Geometry check sheet. Reference: the model listing, model coordinates, mm. Face numbers are marked on the shaded views. A direction names the side the tool comes from. Round coordinates to 2 decimals unless told otherwise and drop trailing zeros. Order: outer loops, then holes, each group sorted by start corner. A loop starts at its lowest first (then second) coordinate and runs counter-clockwise, first axis right, second up.
Autodesk Inventor part; units mm, degrees
ref_plane "Work Plane1" through (-20.5858, -18.5858, -56) normal (0, 0, -1) x (0, 1, 0)
ref_plane "YZ Plane" through (0, 0, 0) normal (1, 0, 0) x (0, 1, 0)
ref_plane "XZ Plane" through (0, 0, 0) normal (0, 1, 0) x (-1, 0, 0)
sketch "Base" plane through (0, 0, 0) normal (0, 0, 1) x (1, 0, 0)
  circle A0 centre (0, 0) radius 11 construction
  line L0 (18, 21) -> (-22, 21) construction
  line L1 (-22, -21) -> (18, -21) construction
  line L2 (19, -20) -> (19, 20) construction
  line L3 (-23, 20) -> (-23, -20) construction
  circle A1 centre (0, 0) radius 11.075
  line L4 (-197.84, 0) -> (55.14, 0) construction
  line L5 (-23, 23.05) -> (19, 23.05)
  line L6 (19, 23.05) -> (19, 21.05)
  line L7 (19, 21.05) -> (-23, 21.05)
  line L8 (-23, 21.05) -> (-23, 23.05)
  line L9 (-23, 21.05) -> (19, 21.05)
  line L10 (19, 21.05) -> (19, 0)
  line L11 (19, 0) -> (-23, 0)
  line L12 (-23, 0) -> (-23, 21.05)
  line L13 (-23, -23.05) -> (19, -23.05)
  line L14 (19, -23.05) -> (19, -21.05)
  line L15 (19, -21.05) -> (-23, -21.05)
  line L16 (-23, -21.05) -> (-23, -23.05)
  line L17 (19, -21.05) -> (19, 0)
  line L18 (-23, 0) -> (-23, -21.05)
  line L19 (0, 14) -> (0, 0) construction
  line L20 (0, 0) -> (0, -14) construction
  circle A2 centre (12.3744, -12.3744) radius 1.621
  circle A3 centre (12.3744, 12.3744) radius 1.621
  circle A4 centre (-12.3744, 12.3744) radius 1.621
  circle A5 centre (-12.3744, -12.3744) radius 1.621
  dimension "d0" = 22.15
  dimension "d1" = 2
  dimension "d4" = 0.05
extrude "BaseFeature" add sketch "Base" along normal blind 4 contours L11 L17 L15 L18 A1 | A1 L11 L12 L7 L10 | L7 L8 L5 L6 | L14 L13 L16 L15
ref_plane "Work Plane1" through (-20.5858, -18.5858, -56) normal (0, 0, -1) x (0, 1, 0)
sketch "Sides" plane through (0, 0, 0) normal (0, 0, -1) x (-1, 0, 0)
  line L0 (23, -23.05) -> (-19, -23.05)
  line L1 (-19, -23.05) -> (23, -23.05)
  line L2 (23, -23.05) -> (23, -21.05)
  line L3 (23, -21.05) -> (-19, -21.05)
  line L4 (-19, -21.05) -> (-19, -23.05)
  line L5 (-19, 23.05) -> (23, 23.05)
  line L6 (-19, 23.05) -> (23, 23.05)
  line L7 (23, 23.05) -> (23, 21.05)
  line L8 (23, 21.05) -> (-19, 21.05)
  line L9 (-19, 21.05) -> (-19, 23.05)
  point P0 (0, 0)
extrude "Extrusion2" add sketch "Sides" along normal blind 8
sketch "Sketch3" plane through (-23, -23.05, 4) normal (0, -1, 0) x (1, 0, 0)
  line L0 (42, -12) -> (42, 0)
  line L1 (0, 0) -> (42, 0)
  line L2 (0, -12) -> (0, 0)
  line L3 (42, -12) -> (0, -12)
  point P0 (23, -4)
extrude "Extrusion3" add sketch "Sketch3" along normal blind 1
mirror "Mirror1" about plane through (0, 0, 0) normal (0, 1, 0) of "Extrusion3"
sketch "Sketch4" plane through (-23, -24.05, 4) normal (0, -1, 0) x (1, 0, 0)
  line L0 (0, 0) -> (0, -12) construction
  line L1 (42, -4) -> (42, -12) construction
  circle A0 centre (5.5, -7.5) radius 1.621
  line L2 (21, 0) -> (21, -12) construction
  line L3 (0, -12) -> (42, -12) construction
  line L4 (42, 0) -> (0, 0) construction
  circle A1 centre (36.5, -7.5) radius 1.621
  point P0 (23, -4)
  dimension "d9" = 3.242
  dimension "d15" = 5.5
  dimension "d16" = 4.5
extrude "Extrusion4" cut sketch "Sketch4" against normal through all
chamfer "Chamfer1" distance 2 angle 45 4 edges at (19, 24.05, -2) (-23, 24.05, -2) (19, -24.05, -2) (-23, -24.05, -2)
properties part number "MotorMount"
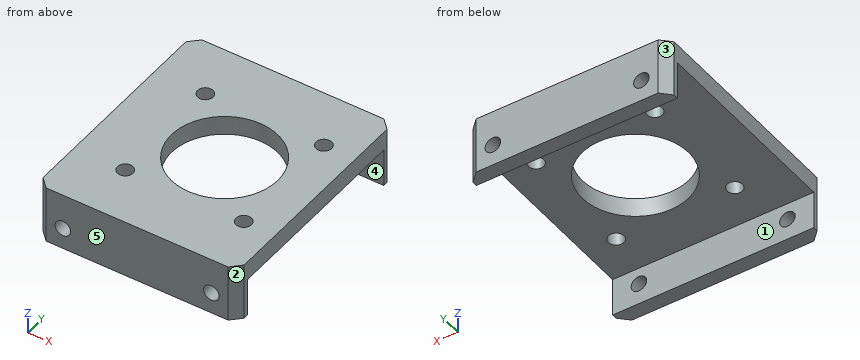
(1) Material ranges on line 1 (Z direction, x = 13.5, y = 22.5); line 2 (Y direction, x = -5, z = -6); line 3 (Z direction, x = 11, y = 9.5), recorded low to high.
Returned:
line 1: z = -8 to -5.12, -1.88 to 4
line 2: y = -24.05 to -21.05, 21.05 to 24.05
line 3: z = 0 to 4
(2) Sectioned sample at A-A, the plane z = -3.5. Record the cut outline in (x, y), and give its area (3 significant figures).
Returned:
outline: (-23, -22.05) - (-21, -24.05) - (-19.12, -24.05) - (-19.12, -21.05) - (-23, -21.05) - close; (-23, 21.05) - (-19.12, 21.05) - (-19.12, 24.05) - (-21, 24.05) - (-23, 22.05) - close; (-15.88, -24.05) - (11.88, -24.05) - (11.88, -21.05) - (-15.88, -21.05) - close; (-15.88, 21.05) - (11.88, 21.05) - (11.88, 24.05) - (-15.88, 24.05) - close; (15.12, -24.05) - (17, -24.05) - (19, -22.05) - (19, -21.05) - (15.12, -21.05) - close; (15.12, 21.05) - (19, 21.05) - (19, 22.05) - (17, 24.05) - (15.12, 24.05) - close
area: 205 mm2
(3) Sectioned sample at D-D, the plane x = -17. Record the cut outline in (y, z).
Returned:
outline: (-24.05, -8) - (-21.05, -8) - (-21.05, -5.04) - (-24.05, -5.04) - close; (-24.05, -1.96) - (-21.05, -1.96) - (-21.05, 0) - (21.05, 0) - (21.05, -1.96) - (24.05, -1.96) - (24.05, 4) - (-24.05, 4) - close; (21.05, -8) - (24.05, -8) - (24.05, -5.04) - (21.05, -5.04) - close
(4) Draft check along Y on the marked faces 3, 4 and 5. Enter one of: released by +Y, released by -Y, zero draft, split by the parting line, or undercut.
Returned:
face 3: released by +Y
face 4: undercut
face 5: released by -Y
(5) Depth check by flat-ended pin: P1, Ø6, axis at x = -11, y = -3, coming from the -Z side. Enter the tip coordinate at first touch or a pass-through.
Returned:
P1: stops at z = 0
(6) Set-up check for the marked faces 1 and 2: record each of +Z, -Z, +X, -X, +Y, -Y from which the full face is reachable in a straight line by a thin tool's end or side.
Returned:
face 1: -Z, +X, -X
face 2: +Z, -Z, +X, -Y
(7) Sectioned sample at B-B, the plane x = 0. Record the cut outline in (y, z) (3 decimals), and give its area (3 significant figures).
Returned:
outline: (-24.05, -8) - (-21.05, -8) - (-21.05, 0) - (-11.075, 0) - (-11.075, 4) - (-24.05, 4) - close; (11.075, 0) - (21.05, 0) - (21.05, -8) - (24.05, -8) - (24.05, 4) - (11.075, 4) - close
area: 152 mm2
(8) Sectioned sample at C-C, the plane y = 0. Record the cut outline in (x, z) (3 decimals), and give its area (3 significant figures).
Returned:
outline: (-23, 0) - (-11.075, 0) - (-11.075, 4) - (-23, 4) - close; (11.075, 0) - (19, 0) - (19, 4) - (11.075, 4) - close
area: 79.4 mm2
